```python
from build123d import *

# Parameters (mm, degrees)
BOSS_EXTRUDE1_DEPTH = 127


with BuildPart() as part:
    # Sketch1 → Boss-Extrude1 (new body)
    with BuildSketch(Plane(origin=(0, 0, -4000), x_dir=(-1, 0, 0), z_dir=(0, 0, -1))):
        with BuildLine():
            Line((10, -8.5), (10, -3.138))
            ThreePointArc((10, -3.138), (9.851210245, -2.778789755), (9.492, -2.63))
            Line((9.492, -2.63), (9.008, -2.63))
            ThreePointArc((9.008, -2.63), (8.648789755, -2.778789755), (8.5, -3.138))
            Line((8.5, -3.138), (8.5, -5.487))
            ThreePointArc((8.5, -5.487), (8.351210245, -5.846210245), (7.992, -5.995))
            Line((7.992, -5.995), (7.26592049, -5.995))
            ThreePointArc((7.26592049, -5.995), (7.071517306, -5.956330803), (6.906710245, -5.846210245))
            Line((6.906710245, -5.846210245), (3.803789755, -2.743289755))
            ThreePointArc((3.803789755, -2.743289755), (3.693669197, -2.578482694), (3.655, -2.38407951))
            Line((3.655, -2.38407951), (3.655, 2.383759167))
            ThreePointArc((3.655, 2.383759167), (3.693669197, 2.57816235), (3.803789755, 2.742969412))
            Line((3.803789755, 2.742969412), (6.907030588, 5.846210245))
            ThreePointArc((6.907030588, 5.846210245), (7.07183765, 5.956330803), (7.266240833, 5.995))
            Line((7.266240833, 5.995), (7.992, 5.995))
            ThreePointArc((7.992, 5.995), (8.351210245, 5.846210245), (8.5, 5.487))
            Line((8.5, 5.487), (8.5, 3.138))
            ThreePointArc((8.5, 3.138), (8.648789755, 2.778789755), (9.008, 2.63))
            Line((9.008, 2.63), (9.492, 2.63))
            ThreePointArc((9.492, 2.63), (9.851210245, 2.778789755), (10, 3.138))
            Line((10, 3.138), (10, 8.5))
            ThreePointArc((10, 8.5), (9.560660172, 9.560660172), (8.5, 10))
            Line((8.5, 10), (3.138, 10))
            ThreePointArc((3.138, 10), (2.778789755, 9.851210245), (2.63, 9.492))
            Line((2.63, 9.492), (2.63, 9.008))
            ThreePointArc((2.63, 9.008), (2.778789755, 8.648789755), (3.138, 8.5))
            Line((3.138, 8.5), (5.487, 8.5))
            ThreePointArc((5.487, 8.5), (5.846210245, 8.351210245), (5.995, 7.992))
            Line((5.995, 7.992), (5.995, 7.26592049))
            ThreePointArc((5.995, 7.26592049), (5.956330803, 7.071517306), (5.846210245, 6.906710245))
            Line((5.846210245, 6.906710245), (2.743289755, 3.803789755))
            ThreePointArc((2.743289755, 3.803789755), (2.578482694, 3.693669197), (2.38407951, 3.655))
            Line((2.38407951, 3.655), (-2.383759167, 3.655))
            ThreePointArc((-2.383759167, 3.655), (-2.57816235, 3.693669197), (-2.742969412, 3.803789755))
            Line((-2.742969412, 3.803789755), (-5.846210245, 6.907030588))
            ThreePointArc((-5.846210245, 6.907030588), (-5.956330803, 7.07183765), (-5.995, 7.266240833))
            Line((-5.995, 7.266240833), (-5.995, 7.992))
            ThreePointArc((-5.995, 7.992), (-5.846210245, 8.351210245), (-5.487, 8.5))
            Line((-5.487, 8.5), (-3.138, 8.5))
            ThreePointArc((-3.138, 8.5), (-2.778789755, 8.648789755), (-2.63, 9.008))
            Line((-2.63, 9.008), (-2.63, 9.492))
            ThreePointArc((-2.63, 9.492), (-2.778789755, 9.851210245), (-3.138, 10))
            Line((-3.138, 10), (-8.5, 10))
            ThreePointArc((-8.5, 10), (-9.560660172, 9.560660172), (-10, 8.5))
            Line((-10, 8.5), (-10, 3.138))
            ThreePointArc((-10, 3.138), (-9.851210245, 2.778789755), (-9.492, 2.63))
            Line((-9.492, 2.63), (-9.008, 2.63))
            ThreePointArc((-9.008, 2.63), (-8.648789755, 2.778789755), (-8.5, 3.138))
            Line((-8.5, 3.138), (-8.5, 5.487))
            ThreePointArc((-8.5, 5.487), (-8.351210245, 5.846210245), (-7.992, 5.995))
            Line((-7.992, 5.995), (-7.26592049, 5.995))
            ThreePointArc((-7.26592049, 5.995), (-7.071517306, 5.956330803), (-6.906710245, 5.846210245))
            Line((-6.906710245, 5.846210245), (-3.803789755, 2.743289755))
            ThreePointArc((-3.803789755, 2.743289755), (-3.693669197, 2.578482694), (-3.655, 2.38407951))
            Line((-3.655, 2.38407951), (-3.655, -2.383759167))
            ThreePointArc((-3.655, -2.383759167), (-3.693669197, -2.57816235), (-3.803789755, -2.742969412))
            Line((-3.803789755, -2.742969412), (-6.907030588, -5.846210245))
            ThreePointArc((-6.907030588, -5.846210245), (-7.07183765, -5.956330803), (-7.266240833, -5.995))
            Line((-7.266240833, -5.995), (-7.992, -5.995))
            ThreePointArc((-7.992, -5.995), (-8.351210245, -5.846210245), (-8.5, -5.487))
            Line((-8.5, -5.487), (-8.5, -3.138))
            ThreePointArc((-8.5, -3.138), (-8.648789755, -2.778789755), (-9.008, -2.63))
            Line((-9.008, -2.63), (-9.492, -2.63))
            ThreePointArc((-9.492, -2.63), (-9.851210245, -2.778789755), (-10, -3.138))
            Line((-10, -3.138), (-10, -8.5))
            ThreePointArc((-10, -8.5), (-9.560660172, -9.560660172), (-8.5, -10))
            Line((-8.5, -10), (-3.138, -10))
            ThreePointArc((-3.138, -10), (-2.778789755, -9.851210245), (-2.63, -9.492))
            Line((-2.63, -9.492), (-2.63, -9.008))
            ThreePointArc((-2.63, -9.008), (-2.778789755, -8.648789755), (-3.138, -8.5))
            Line((-3.138, -8.5), (-5.487, -8.5))
            ThreePointArc((-5.487, -8.5), (-5.846210245, -8.351210245), (-5.995, -7.992))
            Line((-5.995, -7.992), (-5.995, -7.26592049))
            ThreePointArc((-5.995, -7.26592049), (-5.956330803, -7.071517306), (-5.846210245, -6.906710245))
            Line((-5.846210245, -6.906710245), (-2.743289755, -3.803789755))
            ThreePointArc((-2.743289755, -3.803789755), (-2.578482694, -3.693669197), (-2.38407951, -3.655))
            Line((-2.38407951, -3.655), (2.383759167, -3.655))
            ThreePointArc((2.383759167, -3.655), (2.57816235, -3.693669197), (2.742969412, -3.803789755))
            Line((2.742969412, -3.803789755), (5.846210245, -6.907030588))
            ThreePointArc((5.846210245, -6.907030588), (5.956330803, -7.07183765), (5.995, -7.266240833))
            Line((5.995, -7.266240833), (5.995, -7.992))
            ThreePointArc((5.995, -7.992), (5.846210245, -8.351210245), (5.487, -8.5))
            Line((5.487, -8.5), (3.138, -8.5))
            ThreePointArc((3.138, -8.5), (2.778789755, -8.648789755), (2.63, -9.008))
            Line((2.63, -9.008), (2.63, -9.492))
            ThreePointArc((2.63, -9.492), (2.778789755, -9.851210245), (3.138, -10))
            Line((3.138, -10), (8.5, -10))
            ThreePointArc((8.5, -10), (9.560660172, -9.560660172), (10, -8.5))
        make_face()
        with BuildLine():
            Line((2.304493037, -2.124493037), (2.124493037, -2.304493037))
            ThreePointArc((2.124493037, -2.304493037), (1.35638567, -2.506016078), (0.803729988, -1.935777391))
            ThreePointArc((0.803729988, -1.935777391), (0, -2.096), (-0.803729988, -1.935777391))
            ThreePointArc((-0.803729988, -1.935777391), (-1.35638567, -2.506016078), (-2.124493037, -2.304493037))
            Line((-2.124493037, -2.304493037), (-2.304493037, -2.124493037))
            ThreePointArc((-2.304493037, -2.124493037), (-2.506016078, -1.35638567), (-1.935777391, -0.803729988))
            ThreePointArc((-1.935777391, -0.803729988), (-2.096, 0), (-1.935777391, 0.803729988))
            ThreePointArc((-1.935777391, 0.803729988), (-2.506016078, 1.35638567), (-2.304493037, 2.124493037))
            Line((-2.304493037, 2.124493037), (-2.124493037, 2.304493037))
            ThreePointArc((-2.124493037, 2.304493037), (-1.35638567, 2.506016078), (-0.803729988, 1.935777391))
            ThreePointArc((-0.803729988, 1.935777391), (0, 2.096), (0.803729988, 1.935777391))
            ThreePointArc((0.803729988, 1.935777391), (1.35638567, 2.506016078), (2.124493037, 2.304493037))
            Line((2.124493037, 2.304493037), (2.304493037, 2.124493037))
            ThreePointArc((2.304493037, 2.124493037), (2.506016078, 1.35638567), (1.935777391, 0.803729988))
            ThreePointArc((1.935777391, 0.803729988), (2.096, 0), (1.935777391, -0.803729988))
            ThreePointArc((1.935777391, -0.803729988), (2.506016078, -1.35638567), (2.304493037, -2.124493037))
        make_face(mode=Mode.SUBTRACT)
    extrude(amount=-BOSS_EXTRUDE1_DEPTH)


solid = part.part
```
Can you work these out from the model? Positions are in its coordinate system, mm. A direction names the side the tool comes from. Coordinates: 2 decimals unless noted, no trailing zeros.
1) Thinking about a two-plate mould opening in Y: for faces 1 (the flat face through (3.655, 0, -3937)), 2 (the flat face through (-6, -10, -3937)), 3 (the flat face through (10, 6, -3937)), which applies, pulls with the +Y half, pulls with the -Y half, needs draft (parallel to the pull), parting line crosses it, or undercut?
2) I need wall thicknesses on probe 1 along Y at (x, z) = (-1.5, -3970) (3 decimals); probe 2 along Y at (x, z) = (1, -3935) (3 decimals); probe 3 along X at (y, z) = (5.5, -3918). Which ranges of each line are inside material? Lowest first, please.
3) For pin 1 (5 mm diameter, centred on x = 0, z = -3927, fed in from -Y); pin 2 (0.5 mm diameter, centred on x = 9.5, z = -3947, fed in from +Y); pin 3 (4 mm diameter, centred on y = -0.5, z = -3905, fed in from +X), each with a flat end and sliding along its axis, tell me the tip position at first contact or that it passes through.
4) Which directions (+Z, -Z, +X, -X, +Y, -Y) give clear straight access to the entire face, cutting with the end or side of a thin tool? Please do faces 4 (the flat face through (-3.655, 0, -3937)), 5 (the flat face through (4, -8.5, -3937)), 6 (the flat face through (0, 3.655, -3937)), 7 (the flat face through (2.4, 0.1, -3873)), 8 (the flat face through (6, 10, -3937)).
Completed:
1. face 1: undercut
1. face 2: pulls with the -Y half
1. face 3: needs draft
2. probe 1: y = -3.655 to -2.532, 2.532 to 3.655
2. probe 2: y = -3.655 to -2.293, 2.293 to 3.655
2. probe 3: x = -10 to -8.5, -6.56 to -4.44, 4.44 to 6.56, 8.5 to 10
3. pin 1: stops at y = -3.67
3. pin 2: stops at y = 9.8
3. pin 3: stops at x = 3.67
4. face 4: +Z, -Z, -X
4. face 5: +Z, -Z
4. face 6: +Z, -Z, +Y
4. face 7: +Z, +X, -X, +Y, -Y
4. face 8: +Z, -Z, +X, -X, +Y
